from build123d import *

# Parameters (mm, degrees)
REVOLVE1_ANGLE                  = 180
FILLET1_R                       = 3
SKETCH2_W                       = 30
SKETCH2_H                       = 0.5
SKETCH3_R                       = 1.15
CUT_EXTRUDE1_DEPTH              = 5
SKETCH4_W                       = 7
SKETCH4_H                       = 6.3
CUT_EXTRUDE2_DEPTH              = 3.15
CIRPATTERN1_COUNT               = 2
CIRPATTERN1_ANGLE               = 30
CIRPATTERN1_THE_OTHER_WAY_COUNT = 2
CIRPATTERN1_THE_OTHER_WAY_ANGLE = 30
CIRPATTERN2_COUNT               = 2
CIRPATTERN2_ANGLE               = 69


with BuildPart() as part:
    # Sketch1 → Revolve1 (revolve)
    with BuildSketch(Plane.XY):
        Polygon((0, 40), (-27.5, 40), (-22.5, 0), (-18.530888493, 0.496138938), (-22.968871126, 36), (-13, 36), (-13, 28.277027027), (-3, 28.277027027), (-3, 36), (0, 36), align=None)
    revolve(axis=Axis((0, 40, 0), (0, -1, 0)), revolution_arc=REVOLVE1_ANGLE)

    # Fillet1
    fillet1_edges = [part.edges().sort_by_distance(p)[0] for p in [
        (0, 40, -27.5),
    ]]
    fillet(fillet1_edges, radius=FILLET1_R)

    # Sketch2 → Cut-Revolve1 (revolve, cut)
    with BuildSketch(Plane.XY):
        with Locations((1, 32.75)):
            Rectangle(SKETCH2_W, SKETCH2_H)
    revolve(axis=Axis((-14, 32.5, 0), (1, 0, 0)), mode=Mode.SUBTRACT)

    # Sketch3 → Cut-Extrude1 (cut)
    with BuildSketch(Plane.XY):
        with Locations((-24.309743639, 30.602464611)):
            Circle(SKETCH3_R)
        with Locations((-21.033834323, 4.395190082)):
            Circle(SKETCH3_R)
        with Locations((21.033834323, 4.395190082)):
            Circle(SKETCH3_R)
        with Locations((24.309743639, 30.602464611)):
            Circle(SKETCH3_R)
    extrude(amount=-CUT_EXTRUDE1_DEPTH, mode=Mode.SUBTRACT)

    # Sketch4 → Cut-Extrude2 (cut, symmetric)
    with BuildSketch(Plane(origin=(0, 0, 0), x_dir=(0, 0, -1), z_dir=(1, 0, 0))):
        with Locations((22.970533345, 16.85)):
            Rectangle(SKETCH4_W, SKETCH4_H)
    cut_extrude2 = extrude(amount=CUT_EXTRUDE2_DEPTH, both=True, mode=Mode.SUBTRACT)

    # CirPattern1: Cut-Extrude2 ×2 about axis
    cirpattern1_axis = Axis((0, 36.627895796, 0), (0, -1, 0))
    for i in range(1, CIRPATTERN1_COUNT):
        add(cut_extrude2.rotate(cirpattern1_axis, i * CIRPATTERN1_ANGLE / (CIRPATTERN1_COUNT - 1)), mode=Mode.SUBTRACT)

    # CirPattern1 the other way: Cut-Extrude2 ×2 about axis
    cirpattern1_the_other_way_axis = Axis((0, 36.627895796, 0), (0, 1, 0))
    for i in range(1, CIRPATTERN1_THE_OTHER_WAY_COUNT):
        add(cut_extrude2.rotate(cirpattern1_the_other_way_axis, i * CIRPATTERN1_THE_OTHER_WAY_ANGLE / (CIRPATTERN1_THE_OTHER_WAY_COUNT - 1)), mode=Mode.SUBTRACT)

    # CirPattern2: Cut-Extrude2 ×2 about axis
    cirpattern2_axis = Axis((0, 36.627895796, 0), (0, -1, 0))
    for i in range(1, CIRPATTERN2_COUNT):
        add(cut_extrude2.rotate(cirpattern2_axis, i * CIRPATTERN2_ANGLE / (CIRPATTERN2_COUNT - 1)), mode=Mode.SUBTRACT)


solid = part.part
The model under review builds one solid part; all positions refer to its coordinate system, in mm. A direction names the side the tool comes from. Round coordinates to 2 decimals unless told otherwise and drop trailing zeros. Order: outer loops, then holes, each group sorted by start corner. A loop starts at its lowest first (then second) coordinate and runs counter-clockwise, first axis right, second up. Notation, with made-up numbers: (10, 59) -> (54, 59) arc R25 cw to (54, 81) -> close; hole circle Ø5 at (5, 34). An arc over 180 degrees is marked (long way). Use CSV: the item, a comma, the result in double quotes. Start each with the question number.
(1) Consider section B-B on y = 17. Write out the cut boundary in (x, z) (3 decimals), and give its area (3 significant figures).
(2) Wall thickness on probe 1 along X at (y, z) = (34, -5.5); probe 2 along Y at (x, z) = (12.5, -1.5); probe 3 along Z at (x, y) = (6, 34.5): over which ranges is each line inside the solid? List them lowest first. Write a range as from..to.
(3) Mouldability with a two-part tool opening along Z and no side actions: class faces 1 (the face through (0, 28.277, -7)), 2 (the face through (-0.41, 0.47, -18.72)), 3 (the face through (0, 32, -13)) as pulls with the +Z half, pulls with the -Z half, needs draft (parallel to the pull), parting line crosses it, or undercut.
(4) Tool access review of faces 4 (the face through (-21, 4, -5)), 5 (the face through (0, 36, -14)), 6 (the face through (0, 36, -1)), 7 (the face through (-3.15, 17, -22)): name each direction out of +Z, -Z, +X, -X, +Y, -Y from which nothing blocks a thin tool from reaching the whole face with its end or side.
(5) Insertion check: pin 1 (2 mm diameter, centred on x = 8, y = 12, fed in from +Z); pin 2 (1.4 mm diameter, centred on x = 24.31, y = 30.6, fed in from -Z); pin 3 (4 mm diameter, centred on y = 8, z = -20.5, fed in from -X). Each pin has a flat end and moves straight along its axis. Give the tip position at first contact, or say it passes through.
(6) Consider section C-C on z = -2. State how many separate pieces and enclosed holes the cut face has, and give its area (3 significant figures).
(7) Consider section A-A on x = 0. Write out the cut boundary in (y, z), and give its area (3 significant figures).
(8) Consider section D-D on y = 8. Write out the cut boundary in (x, z).
Responses:
1,outline,"(-24.625, 0) arc R24.625 ccw to (-14.939, -19.576) -> (-12.904, -16.05) arc R20.594 cw to (-20.594, 0) -> close; (-9.483, -22.726) arc R24.625 ccw to (-3.15, -24.423) -> (-3.15, -20.352) arc R20.594 cw to (-7.448, -19.2) -> close; (3.15, -24.423) arc R24.625 ccw to (9.483, -22.726) -> (7.448, -19.2) arc R20.594 cw to (3.15, -20.352) -> close; (12.904, -16.05) -> (14.939, -19.576) arc R24.625 ccw to (21.672, -11.693) -> (17.871, -10.234) arc R20.594 cw to start; (20.129, -4.353) -> (23.929, -5.812) arc R24.625 ccw to (24.625, 0) -> (20.594, 0) arc R20.594 cw to start"
1,area,"184 mm²"
2,probe 1,"-26.18..-22.04, -11.78..11.78, 22.04..26.18"
2,probe 2,"28.28..40"
2,probe 3,"-26.13..-21.98, -11.53..0"
3,face 1,"needs draft"
3,face 2,"pulls with the +Z half"
3,face 3,"undercut"
4,face 4,"+Z"
4,face 5,"none"
4,face 6,"+Z, -Y"
4,face 7,"+Z, -Z"
5,pin 1,"z = -17.81"
5,pin 2,"z = -11.66"
5,pin 3,"x = -14.52"
6,separate pieces,"1"
6,enclosed holes,"4"
6,area,"649 mm²"
7,outline,"(0, -22.5) -> (13.7, -24.21) -> (13.7, -20.18) -> (0.5, -18.53) -> close; (20, -25) -> (36.63, -27.08) arc R3 ccw to (40, -24.1) -> (40, 0) -> (36, 0) -> (36, -3) -> (28.28, -3) -> (28.28, -13) -> (36, -13) -> (36, -22.97) -> (20, -20.97) -> close"
7,area,"302 mm²"
8,outline,"(-23.5, 0) arc R23.5 ccw to (23.5, 0) -> (19.47, 0) arc R19.47 cw to (-19.47, 0) -> close"
